Model file for the job. Use its own axes, mm. Face numbers are marked on the shaded views. A direction names the side the tool comes from. Round coordinates to 2 decimals unless told otherwise and drop trailing zeros. Order: outer loops, then holes, each group sorted by start corner. A loop starts at its lowest first (then second) coordinate and runs counter-clockwise, first axis right, second up. Notation, with made-up numbers: (16.5, 38) - (46.5, 38) arc R9 cw to (46.5, 46) - close; hole circle Ø7 at (-3, 64). An arc over 180 degrees is marked (long way). Put each result on its own line as item: value. Start each with the question number.
Item 1: Probe probe 1 along Z at (x, y) = (-3.25, 4); probe 2 along Z at (x, y) = (3.5, -1.7); probe 3 along X at (y, z) = (-1.5, -72.25). List the from-to ranges inside material, lowest first.
Item 2: Saw through at A-A on z = -72.25. List the corners of the cut face in (x, y), plus the area to 3 significant figures.
Item 3: Pin check, flat tips, straight feed: pin 1 Ø1 at (x, z) = (-1, -17.5) entering from +Y; pin 2 Ø12 at (x, z) = (4.5, -78.5) entering from +Y; pin 3 Ø4 at (x, z) = (9, -54) entering from +Y; pin 4 Ø2 at (x, y) = (0.5, 3) entering from +Z. Stop position of each tip, or through.
Item 4: Which spindle directions (+Z, -Z, +X, -X, +Y, -Y) get a long thin tool onto all of the face, cutting with end or side? Do the marked faces 1 and 2. Say none if no direction does.
Item 5: Saw through at D-D on z = -86.5. List the corners of the cut face in (x, y).
Item 6: Saw through at C-C on z = -19.75. List the corners of the cut face in (x, y), plus the area to 3 significant figures.
Item 7: Saw through at B-B on x = 3.5. List the corners of the cut face in (y, z), plus the area to 3 significant figures.
```python
from build123d import *

# Parameters (mm, degrees)
SKETCH_1_W                     = 9.5
SKETCH_1_H                     = 13.25
EXTRUDE_1_DEPTH                = 2
EXTRUDE_2_DEPTH                = 12
PATTERN_LINEAR_1_COUNT         = 5
PATTERN_LINEAR_1_PITCH         = 22
HOLE_WIZARD_2_2_2_2_1_D        = 2.1
EXTRUDE_3_DEPTH                = 12
SKETCH_7_W                     = 1.05
SKETCH_7_H                     = 15
EXTRUDE_4_DEPTH                = 110
SKETCH_13_W                    = 1
SKETCH_13_H                    = 38.681287062
HOLE_WIZARD_2_0_2_2_AT_2_COUNT = 2
HOLE_WIZARD_2_0_2_2_AT_2_PITCH = 47
CUT_EXTRUDE_1_DEPTH            = 140.431241936
CUT_EXTRUDE_1_DEPTH_BACK       = 140.431241936
SKETCH_14_W                    = 52.846717088
SKETCH_14_H                    = 8
EXTRUDE23_DEPTH                = 109
EXTRUDE23_DEPTH_BACK           = 77
SKETCH18_W                     = 126.116691802
SKETCH18_H                     = 130.968537131
SKETCH20_W                     = 20
SKETCH20_H                     = 100
EXTRUDE24_DEPTH                = 2
SKETCH21_R                     = 1.1
EXTRUDE25_DEPTH                = 2
EXTRUDE26_DEPTH                = 136
EXTRUDE26_DEPTH_BACK           = 62
SKETCH22_W                     = 135.680863596
SKETCH22_H                     = 114.529775135
SKETCH_15_W                    = 16.5
SKETCH_15_H                    = 100
CUT_EXTRUDE_2_DEPTH            = 1
SKETCH_16_W                    = 20
SKETCH_16_H                    = 100
SKETCH_16_R                    = 1.1
EXTRUDE_5_DEPTH                = 1


with BuildPart() as part:
    # 草图1 → 凸台-拉伸1 (new body)
    with BuildSketch(Plane(origin=(0, 0, 0), x_dir=(1, 0, 0), z_dir=(0, 1, 0))):
        Polygon((21.5, 0), (21.5, 110), (9, 110), (0, 101), (0, 0), align=None)
        Polygon((19.121320344, 101), (4.242640687, 101), (8.121320344, 104.878679656), (19.121320344, 104.878679656), align=None, mode=Mode.SUBTRACT)
        with Locations((10.75, 12.625)):
            Rectangle(SKETCH_1_W, SKETCH_1_H, mode=Mode.SUBTRACT)
        with Locations((10.75, 37.875)):
            Rectangle(SKETCH_1_W, SKETCH_1_H, mode=Mode.SUBTRACT)
        with Locations((10.75, 63.125)):
            Rectangle(SKETCH_1_W, SKETCH_1_H, mode=Mode.SUBTRACT)
        with Locations((10.75, 88.375)):
            Rectangle(SKETCH_1_W, SKETCH_1_H, mode=Mode.SUBTRACT)
    extrude(amount=EXTRUDE_1_DEPTH)

    # 草图2 → 凸台-拉伸2 (add)
    with BuildSketch(Plane(origin=(0, 0, -101), x_dir=(-1, 0, 0), z_dir=(0, 0, -1))):
        with BuildLine():
            Line((0, 2), (0, 0))
            Line((0, 0), (3.5, 0))
            ThreePointArc((3.5, 0), (5.08113883, 4.436491673), (1.050510257, 2))
            Line((1.050510257, 2), (0, 2))
        make_face()
    extrude_2 = extrude(amount=-EXTRUDE_2_DEPTH)

    # 阵列(线性)1: 凸台-拉伸2 ×5
    with Locations(*[(0, 0, i * PATTERN_LINEAR_1_PITCH) for i in range(1, PATTERN_LINEAR_1_COUNT)]):
        add(extrude_2)

    # Ø2.2 (2.2) 直径孔1 (through all)
    with Locations(Plane(origin=(0, 0, -101), x_dir=(-1, 0, 0), z_dir=(0, 0, -1))):
        with Locations((3.5, 2.5)):
            Hole(HOLE_WIZARD_2_2_2_2_1_D / 2)

    # 草图8 → 凸台-拉伸4 (add)
    with BuildSketch(Plane.XY):
        with BuildLine():
            ThreePointArc((31.5, 0), (34.178784027, 0.532843272), (36.449747468, 2.050252532))
            Line((36.449747468, 2.050252532), (39.577164466, 5.17766953))
            ThreePointArc((39.577164466, 5.17766953), (57.254833996, 12.5), (74.932503526, 5.17766953))
            Line((74.932503526, 5.17766953), (76.346717088, 6.591883092))
            ThreePointArc((76.346717088, 6.591883092), (57.254833996, 14.5), (38.162950904, 6.591883092))
            Line((38.162950904, 6.591883092), (35.035533906, 3.464466094))
            ThreePointArc((35.035533906, 3.464466094), (33.413417162, 2.380602337), (31.5, 2))
            Line((31.5, 2), (21.5, 2))
            Line((21.5, 2), (21.5, 0))
            Line((21.5, 0), (31.5, 0))
        make_face()
    extrude(amount=-EXTRUDE_4_DEPTH)

    # 草图13 → Ø2.0 (2) 直径孔2 (revolve, cut)
    with BuildSketch(Plane(origin=(66.489377866, 12.871700761, -5), x_dir=(-0.9396926207859126, 0.34202014332565694, 0), z_dir=(0, 0, 1))):
        with Locations((0.5, 19.340643531)):
            Rectangle(SKETCH_13_W, SKETCH_13_H)
    hole_wizard_2_0_2_2 = revolve(axis=Axis((68.661205776, 18.838748903, -5), (-0.3420201433256569, -0.9396926207859128, 0)), mode=Mode.SUBTRACT)

    # Ø2.0 (2) 直径孔2 at 2: Ø2.0 (2) 直径孔2 ×2
    with Locations(*[(0, 0, -i * HOLE_WIZARD_2_0_2_2_AT_2_PITCH) for i in range(1, HOLE_WIZARD_2_0_2_2_AT_2_COUNT)]):
        add(hole_wizard_2_0_2_2, mode=Mode.SUBTRACT)

    # 草图14 → 切除-拉伸1 (cut, two sides: drawn at the far end of the back side and taken through both)
    with BuildSketch(Plane(origin=(0, 2, 0), x_dir=(1, 0, 0), z_dir=(0, 1, 0)).offset(-CUT_EXTRUDE_1_DEPTH_BACK)):
        with BuildLine():
            add(Edge.make_bspline(
                [(65.543349365, 52), (65.543349365, 51.867858182), (65.568139282, 51.738193315), (65.663651177, 51.49599396), (65.734288369, 51.385069362), (65.909329104, 51.20058787), (66.014984918, 51.126085586), (66.242291721, 51.026337096), (66.366299142, 51.000069682), (66.611454679, 50.999930602), (66.734292904, 51.025809235), (66.960669981, 51.125923854), (67.063423157, 51.199243917), (67.237262204, 51.385832013), (67.305425299, 51.495895945), (67.398649167, 51.738239585), (67.422691544, 51.869119898), (67.422777552, 52.130169285), (67.398544475, 52.261724961), (67.306168595, 52.502477284), (67.237041074, 52.614131138), (67.065581718, 52.798710334), (66.962099904, 52.873181003), (66.736029766, 52.973681753), (66.61428089, 52.999865952), (66.366377399, 53.000133023), (66.24402893, 52.974291959), (66.014886358, 52.874003493), (65.90992169, 52.799906628), (65.647004042, 52.52319771), (65.543349365, 52.264283637), (65.543349365, 52)],
                knots=[0, 0, 0, 0, 0.0625, 0.0625, 0.125, 0.125, 0.1875, 0.1875, 0.25, 0.25, 0.3125, 0.3125, 0.375, 0.375, 0.4375, 0.4375, 0.5, 0.5, 0.5625, 0.5625, 0.625, 0.625, 0.6875, 0.6875, 0.75, 0.75, 0.8125, 0.8125, 0.875, 0.875, 1, 1, 1, 1], degree=3))
        make_face()
        with BuildLine():
            add(Edge.make_bspline(
                [(65.543349365, 5), (65.543349365, 4.867858182), (65.568139282, 4.738193315), (65.663651177, 4.49599396), (65.734288369, 4.385069362), (65.909329104, 4.20058787), (66.014984918, 4.126085586), (66.242291721, 4.026337096), (66.366299142, 4.000069682), (66.611454679, 3.999930602), (66.734292904, 4.025809235), (66.960669981, 4.125923854), (67.063423157, 4.199243917), (67.237262204, 4.385832013), (67.305425299, 4.495895945), (67.398649167, 4.738239585), (67.422691544, 4.869119898), (67.422777552, 5.130169285), (67.398544475, 5.261724961), (67.306168595, 5.502477284), (67.237041074, 5.614131138), (67.065581718, 5.798710334), (66.962099904, 5.873181003), (66.736029766, 5.973681753), (66.61428089, 5.999865952), (66.366377399, 6.000133023), (66.24402893, 5.974291959), (66.014886358, 5.874003493), (65.90992169, 5.799906628), (65.647004042, 5.52319771), (65.543349365, 5.264283637), (65.543349365, 5)],
                knots=[0, 0, 0, 0, 0.0625, 0.0625, 0.125, 0.125, 0.1875, 0.1875, 0.25, 0.25, 0.3125, 0.3125, 0.375, 0.375, 0.4375, 0.4375, 0.5, 0.5, 0.5625, 0.5625, 0.625, 0.625, 0.6875, 0.6875, 0.75, 0.75, 0.8125, 0.8125, 0.875, 0.875, 1, 1, 1, 1], degree=3))
        make_face()
        with Locations((46.923358544, 14)):
            Rectangle(SKETCH_14_W, SKETCH_14_H)
        with Locations((46.923358544, 61)):
            Rectangle(SKETCH_14_W, SKETCH_14_H)
    extrude(amount=CUT_EXTRUDE_1_DEPTH + CUT_EXTRUDE_1_DEPTH_BACK, mode=Mode.SUBTRACT)

    # Sketch18 → Extrude23 (cut, two sides: drawn at the far end of the back side and taken through both)
    with BuildSketch(Plane(origin=(0, 2, 0), x_dir=(1, 0, 0), z_dir=(0, 1, 0)).offset(-EXTRUDE23_DEPTH_BACK)):
        with Locations((63.058345901, 59.008314148)):
            Rectangle(SKETCH18_W, SKETCH18_H)
    extrude(amount=EXTRUDE23_DEPTH + EXTRUDE23_DEPTH_BACK, mode=Mode.SUBTRACT)


with BuildPart() as body_2:
    # 草图5 → 凸台-拉伸3 (new body)
    with BuildSketch(Plane(origin=(9, 0, 0), x_dir=(0, 0, -1), z_dir=(1, 0, 0))):
        with BuildLine():
            Line((-111.050510257, 0), (-109.949581771, 0))
            Line((-109.949581771, 0), (-109.949581771, 2))
            Line((-109.949581771, 2), (-113.5, 2))
            ThreePointArc((-113.5, 2), (-115.08113883, -2.436491673), (-111.050510257, 0))
        make_face()
    extrude(amount=-EXTRUDE_3_DEPTH)

    # 草图7 → Ø2.2 (2.2) 直径孔2 (revolve, cut)
    with BuildSketch(Plane(origin=(9, -0.5, 113.5), x_dir=(0, 0, -1), z_dir=(0, 1, 0))):
        with Locations((0.525, 7.5)):
            Rectangle(SKETCH_7_W, SKETCH_7_H)
    revolve(axis=Axis((15.35, -0.5, 113.5), (-1, 0, 0)), mode=Mode.SUBTRACT)

    # Sketch22 → Extrude26 (cut, two sides: drawn at the far end of the back side and taken through both)
    with BuildSketch(Plane(origin=(0, 0, 0), x_dir=(1, 0, 0), z_dir=(0, 1, 0)).offset(-EXTRUDE26_DEPTH_BACK)):
        with Locations((8.341327017, -106.523866824)):
            Rectangle(SKETCH22_W, SKETCH22_H)
    extrude(amount=EXTRUDE26_DEPTH + EXTRUDE26_DEPTH_BACK, mode=Mode.SUBTRACT)


with BuildPart() as extrude23_piece_1:
    # of the separate pieces the step leaves, piece 1, a body of its own (extrude23_pieces)
    add(part.part.solids().sort_by_distance((0, 2, -101))[0])



with BuildPart() as extrude23_piece_2:
    # of the separate pieces the step leaves, piece 2, a body of its own (extrude23_pieces)
    add(part.part.solids().sort_by_distance((0, 2, -79))[0])


with BuildPart() as extrude23_piece_3:
    # of the separate pieces the step leaves, piece 3, a body of its own (extrude23_pieces)
    add(part.part.solids().sort_by_distance((0, 2, -57))[0])


with BuildPart() as extrude23_piece_4:
    # of the separate pieces the step leaves, piece 4, a body of its own (extrude23_pieces)
    add(part.part.solids().sort_by_distance((0, 2, -35))[0])


with BuildPart() as extrude23_piece_5:
    # of the separate pieces the step leaves, piece 5, a body of its own (extrude23_pieces)
    add(part.part.solids().sort_by_distance((-1.050510257, 2, -1))[0])


with BuildPart() as extrude23_piece_1_1:
    add(extrude23_piece_1.part)

    add(extrude23_piece_2.part)  # Extrude24 merges Extrude23 piece 2

    add(extrude23_piece_3.part)  # Extrude24 merges Extrude23 piece 3

    add(extrude23_piece_4.part)  # Extrude24 merges Extrude23 piece 4

    add(extrude23_piece_5.part)  # Extrude24 merges Extrude23 piece 5
    # Sketch20 → Extrude24 (add)
    with BuildSketch(Plane(origin=(0, 0, 0), x_dir=(-1, 0, 0), z_dir=(0, -1, 0))):
        with Locations((-6.5, 51)):
            Rectangle(SKETCH20_W, SKETCH20_H)
    extrude(amount=EXTRUDE24_DEPTH)

    # Sketch21 → Extrude25 (cut)
    with BuildSketch(Plane(origin=(0, 0, 0), x_dir=(1, 0, 0), z_dir=(0, 1, 0))):
        with Locations(Location((3.5, 89.25, 0), (0, 0, 270))):
            Circle(SKETCH21_R)
        with Locations(Location((3.5, 72.25, 0), (0, 0, 270))):
            Circle(SKETCH21_R)
        with Locations(Location((3.5, 36.75, 0), (0, 0, 270))):
            Circle(SKETCH21_R)
        with Locations(Location((3.5, 19.75, 0), (0, 0, 270))):
            Circle(SKETCH21_R)
    extrude(amount=-EXTRUDE25_DEPTH, mode=Mode.SUBTRACT)

    # 草图15 → 切除-拉伸2 (cut)
    with BuildSketch(Plane(origin=(0, 0, 0), x_dir=(1, 0, 0), z_dir=(0, 1, 0))):
        with Locations((8.25, 51)):
            Rectangle(SKETCH_15_W, SKETCH_15_H)
    extrude(amount=-CUT_EXTRUDE_2_DEPTH, mode=Mode.SUBTRACT)

    # 草图16 → 凸台-拉伸5 (add)
    with BuildSketch(Plane(origin=(0, -2, 0), x_dir=(-1, 0, 0), z_dir=(0, -1, 0))):
        with Locations((-6.5, 51)):
            Rectangle(SKETCH_16_W, SKETCH_16_H)
        with Locations(Location((-3.5, 89.25, 0), (0, 0, 270))):
            Circle(SKETCH_16_R, mode=Mode.SUBTRACT)
        with Locations(Location((-3.5, 72.25, 0), (0, 0, 270))):
            Circle(SKETCH_16_R, mode=Mode.SUBTRACT)
        with Locations(Location((-3.5, 36.75, 0), (0, 0, 270))):
            Circle(SKETCH_16_R, mode=Mode.SUBTRACT)
        with Locations(Location((-3.5, 19.75, 0), (0, 0, 270))):
            Circle(SKETCH_16_R, mode=Mode.SUBTRACT)
    extrude(amount=EXTRUDE_5_DEPTH)


solid = extrude23_piece_1_1.part
```
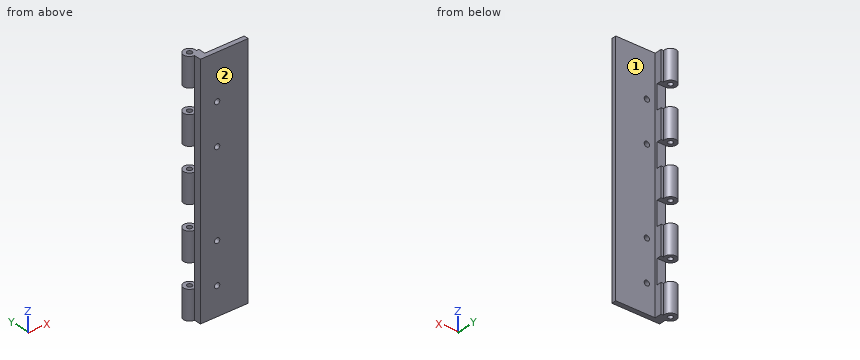
Results found:
1. probe 1: z = -101 to -89, -79 to -67, -57 to -45, -35 to -23, -13 to -1
1. probe 2: z = -101 to -90.35, -88.15 to -73.35, -71.15 to -37.85, -35.65 to -20.85, -18.65 to -1
1. probe 3: x = -3.5 to 2.4, 4.6 to 16.5
2. outline: (-3.5, -3) - (2.4, -3) - (2.4, -1) - (0, -1) - (0, 2) - (-1.05, 2) arc R2.5 ccw (long way) to (-3.5, 0) - close; (4.6, -3) - (16.5, -3) - (16.5, -1) - (4.6, -1) - close; hole circle Ø2.1 at (-3.5, 2.5)
2. area: 58.6 mm²
3. pin 1: stops at y = 0
3. pin 2: stops at y = 4
3. pin 3: stops at y = -1
3. pin 4: passes through
4. face 1: +Z, -Z, +X, +Y
4. face 2: +Z, -Z, +X, -X, -Y
5. outline: (-3.5, -3) - (16.5, -3) - (16.5, -1) - (0, -1) - (0, 0) - (-3.5, 0) - close
6. outline: (-3.5, -3) - (2.4, -3) - (2.4, -1) - (0, -1) - (0, 0) - (-3.5, 0) - close; (4.6, -3) - (16.5, -3) - (16.5, -1) - (4.6, -1) - close
6. area: 39.1 mm²
7. outline: (-3, -101) - (-1, -101) - (-1, -90.35) - (-3, -90.35) - close; (-3, -88.15) - (-1, -88.15) - (-1, -73.35) - (-3, -73.35) - close; (-3, -71.15) - (-1, -71.15) - (-1, -37.85) - (-3, -37.85) - close; (-3, -35.65) - (-1, -35.65) - (-1, -20.85) - (-3, -20.85) - close; (-3, -18.65) - (-1, -18.65) - (-1, -1) - (-3, -1) - close
7. area: 182 mm²
